Read the model definition and answer for the solid it produces. Units are mm, in the model's axes. Give positions to 0.01 mm unless a question says otherwise; leave off trailing zeros. Write each loop counter-clockwise with the first axis right and the second up, starting at its lowest first coordinate (ties: lowest second). Pieces come first, ordered by that corner, then holes. Notation, with made-up numbers: M 71,56.25 L 115,56.25 A21 cw 115,91.25 Z; hole C 67.5,-30 d9. An arc over 180 degrees is marked long. Put each result on its own line as item: value.
Autodesk Inventor part; units mm, degrees
ref_plane "YZ Plane" through (0, 0, 0) normal (1, 0, 0) x (0, 1, 0)
ref_plane "XZ Plane" through (0, 0, 0) normal (0, 1, 0) x (-1, 0, 0)
ref_plane "XY Plane" through (0, 0, 0) normal (0, 0, 1) x (1, 0, 0)
sketch "Sketch1" plane through (0, 0, 0) normal (1, 0, 0) x (0, 1, 0)
  circle A0 centre (0, 0) radius 57.3659
  circle A1 centre (0, 0) radius 37.4904
  circle A2 centre (26.5097, 26.5097) radius 6.985
  line L0 (0, 0) -> (26.5097, 26.5097)
  line L1 (0, 0) -> (37.4904, 0) construction
  circle A3 centre (-9.7032, 36.2129) radius 6.985
  circle A4 centre (-36.2129, 9.7032) radius 6.985
  circle A5 centre (-26.5097, -26.5097) radius 6.985
  circle A6 centre (9.7032, -36.2129) radius 6.985
  circle A7 centre (36.2129, -9.7032) radius 6.985
  circle A8 centre (0, 0) radius 15.875
  circle A9 centre (60.1365, 16.1135) radius 15.875
  line L2 (0, 0) -> (62.2818, 0) construction
  line L3 (0, 0) -> (54.4204, 0) construction
  line L4 (0, 0) -> (47.0027, 0) construction
  line L5 (0, 0) -> (74.4134, 19.939)
  line L6 (0, 0) -> (77.0384, 0) construction
  circle A10 centre (0, 0) radius 15.875
  circle A11 centre (16.1135, 60.1365) radius 15.875
  circle A12 centre (0, 0) radius 15.875
  circle A13 centre (-44.023, 44.023) radius 15.875
  circle A14 centre (0, 0) radius 15.875
  circle A15 centre (-60.1365, -16.1135) radius 15.875
  circle A16 centre (0, 0) radius 15.875
  circle A17 centre (-16.1135, -60.1365) radius 15.875
  circle A18 centre (0, 0) radius 15.875
  circle A19 centre (44.023, -44.023) radius 15.875
  line L7 (0, 0) -> (-9.7032, 36.2129)
  line L8 (0, 0) -> (-36.2129, 9.7032)
  point P0 (36.2129, 9.7032)
  point P1 (49.9198, 28.264)
  point P2 (28.264, 49.9198)
  point P3 (0.4825, 57.3639)
  point P4 (-29.0998, 49.4373)
  point P5 (-49.4373, 29.0998)
  point P6 (-57.3639, -0.4825)
  point P7 (-49.9198, -28.264)
  point P8 (-28.264, -49.9198)
  point P9 (-0.4825, -57.3639)
  point P10 (29.0998, -49.4373)
  point P11 (49.4373, -29.0998)
  point P12 (57.3639, 0.4825)
  dimension "d0" = 114.7318
  dimension "d1" = 74.9808
  dimension "d2" = 13.97
  dimension "d3" = 45
  dimension "d6" = 360
  dimension "d8" = 31.75
  dimension "d12" = 31.75
  dimension "d16" = 15
  dimension "d19" = 360
  dimension "d24" = 21.6154
  dimension "d25" = 60.1365
extrude "Extrusion1" add sketch "Sketch1" along normal blind 7.9375 contours A1 A7 A6 A5 A4 L8 A8 L5 | L5 A8 L0 A2 A1 | A0 A19 A17 A15 A13 A11 A9 | L0 A8 L7 A3 A1 A2 | L8 A4 A1 A3 L7 A8
fillet "Fillet1" radius 3.175 12 edges at (3.9688, 57.3639, 0.4825) (3.9688, 49.9198, 28.264) (3.9688, 29.0998, -49.4373) (3.9688, 49.4373, -29.0998) (3.9688, -0.4825, -57.3639) (3.9688, -28.264, -49.9198) (3.9688, -49.9198, -28.264) (3.9688, -57.3639, -0.4825) (3.9688, -49.4373, 29.0998) (3.9688, -29.0998, 49.4373) (3.9688, 0.4825, 57.3639) (3.9688, 28.264, 49.9198)
properties part number "DTR-4"
(1) Section C-C on z = -14 is taken. Determine the outline of the cut face in (x, y), and give its area (3 significant figures).
Result:
outline: M 0,-44.4 L 7.94,-44.4 L 7.94,-7.48 L 0,-7.48 Z; M 0,7.48 L 7.94,7.48 L 7.94,30.71 L 0,30.71 Z; M 0,41.72 L 7.94,41.72 L 7.94,55.63 L 0,55.63 Z
area: 588 mm²
(2) Given pin 1 Ø1 at (x, z) = (7, -21.5) entering from -Y; pin 2 Ø1 at (x, y) = (4.5, -38) entering from +Z; pin 3 Ø3 at (x, y) = (2, -35.5) entering from -Z; pin 4 Ø16 at (y, z) = (-36.21, 9.7) entering from +X, each flat-ended and moving along its own axis, determine where each tip first touches the part or whether it passes through.
Result:
pin 1: stops at y = -45.39
pin 2: stops at z = 29.55
pin 3: stops at z = -46.2
pin 4: stops at x = 7.94
(3) For a pull along Y with two mould halves and no side action, classify faces 1 (the face through (3.913, -12.218, -44.747)), 2 (the face through (3.913, 15.022, -55.364)), 3 (the face through (3.913, -15.022, 55.364)) as +Y half, -Y half, draft (parallel to the pull), parting line (faces both ways), or undercut.
Result:
face 1: undercut
face 2: +Y half
face 3: -Y half
(4) Straight lines are drawn through the part: line 1 along Z through (x, y) = (7, 12); line 2 along Z through (x, y) = (5.25, 9); line 3 along Y through (x, z) = (4.75, -5.5). For each, find the intervals that lie inside material, in ascending order. Write a range as from..to.
Result:
line 1: z = -56.1..-42.81, -29.62..-10.39, 10.39..44.8
line 2: z = -56.66..-43.16, -29.26..-13.08, 13.08..45.94
line 3: y = -48.33..-14.89, 14.89..30.63, 41.79..57.1
(5) Section D-D on x = 6 is taken. Give the number of separate pieces and of enclosed holes in the cut face, and give its area (3 significant figures).
Result:
separate pieces: 1
enclosed holes: 7
area: 7,270 mm²
(6) Section B-B on z = 22 is taken. Determine the outline of the cut face in (x, y).
Result:
outline: M 0,-52.98 L 7.94,-52.98 L 7.94,21.18 L 0,21.18 Z; M 0,31.84 L 7.94,31.84 L 7.94,45.39 L 0,45.39 Z
(7) Section A-A on y = 9 is taken. Determine the outline of the cut face in (x, z), and give its area (3 significant figures).
Result:
outline: M 0,-56.66 L 7.94,-56.66 L 7.94,-43.16 L 0,-43.16 Z; M 0,-29.26 L 7.94,-29.26 L 7.94,-13.08 L 0,-13.08 Z; M 0,13.08 L 7.94,13.08 L 7.94,45.94 L 0,45.94 Z
area: 496 mm²
